from build123d import *

# Parameters (mm, degrees)
SKETCH1_R                 = 31.75
CENTERCIRCLEEXTRUDE_DEPTH = 19.558
SKETCH2_R                 = 80.01
BASEEXPAND_DEPTH          = 7.62
SKETCH3_R                 = 27.559
CENTERCUT_DEPTH           = 27.178
SKETCH4_R                 = 6.731
OUTERCIRCLECUT_DEPTH      = 7.62
SKETCH8_R                 = 80.01
STARFISHCUT_DEPTH         = 7.62
BATMAN_CUT_DEPTH          = 5.08
FILLET1_R                 = 2.54


with BuildPart() as part:
    # Sketch1 → CenterCircleExtrude (new body)
    with BuildSketch(Plane(origin=(0, 0, 0), x_dir=(1, 0, 0), z_dir=(0, 1, 0))):
        with Locations(Location((0, 0, 0), (0, 0, 270))):
            Circle(SKETCH1_R)
    extrude(amount=CENTERCIRCLEEXTRUDE_DEPTH)

    # Sketch2 → BaseExpand (add)
    with BuildSketch(Plane.XZ):
        with Locations(Location((0, 0, 0), (0, 0, 90))):
            Circle(SKETCH2_R)
    extrude(amount=BASEEXPAND_DEPTH)

    # Sketch3 → CenterCut (cut)
    with BuildSketch(Plane(origin=(0, 19.558, 0), x_dir=(1, 0, 0), z_dir=(0, 1, 0))):
        with Locations(Location((0, 0, 0), (0, 0, 270))):
            Circle(SKETCH3_R)
    extrude(amount=-CENTERCUT_DEPTH, mode=Mode.SUBTRACT)

    # Sketch4 → OuterCircleCut (cut)
    with BuildSketch(Plane(origin=(0, 0, 0), x_dir=(1, 0, 0), z_dir=(0, 1, 0))):
        with Locations(Location((-0.261130397, 55.117381423, 0), (0, 0, 270))):
            Circle(SKETCH4_R)
        with Locations(Location((47.602487304, 27.784836269, 0), (0, 0, 270))):
            Circle(SKETCH4_R)
        with Locations(Location((47.863617701, -27.332545154, 0), (0, 0, 270))):
            Circle(SKETCH4_R)
        with Locations(Location((0.261130397, -55.117381423, 0), (0, 0, 270))):
            Circle(SKETCH4_R)
        with Locations(Location((-47.602487304, -27.784836269, 0), (0, 0, 270))):
            Circle(SKETCH4_R)
        with Locations(Location((-47.863617701, 27.332545154, 0), (0, 0, 270))):
            Circle(SKETCH4_R)
    extrude(amount=-OUTERCIRCLECUT_DEPTH, mode=Mode.SUBTRACT)

    # Sketch8 → StarfishCut (cut)
    with BuildSketch(Plane(origin=(0, 0, 0), x_dir=(1, 0, 0), z_dir=(0, 1, 0))):
        Circle(SKETCH8_R)
        with BuildLine():
            ThreePointArc((-9.691634922, 58.167231466), (0, 65.278), (9.691634922, 58.167231466))
            ThreePointArc((9.691634922, 58.167231466), (14.680421474, 46.487646722), (20.366200635, 35.131036031))
            ThreePointArc((20.366200635, 35.131036031), (32.932591729, 35.888695551), (45.430991402, 37.398079103))
            ThreePointArc((45.430991402, 37.398079103), (46.084351809, 37.521062437), (46.744356679, 37.60105177))
            ThreePointArc((46.744356679, 37.60105177), (54.497784748, 34.973113956), (57.796096952, 27.480261323))
            ThreePointArc((57.796096952, 27.480261323), (57.324919213, 24.422104494), (55.95508845, 21.647596369))
            ThreePointArc((55.95508845, 21.647596369), (55.55581322, 21.116010052), (55.122626325, 20.611675009))
            ThreePointArc((55.122626325, 20.611675009), (47.502202506, 10.451466749), (40.509978727, -0.15086779))
            ThreePointArc((40.509978727, -0.15086779), (47.449326667, -10.654851952), (55.005691003, -20.7240918))
            ThreePointArc((55.005691003, -20.7240918), (55.438877898, -21.228426843), (55.838153128, -21.76001316))
            ThreePointArc((55.838153128, -21.76001316), (57.207983891, -24.534521285), (57.67916163, -27.592678114))
            ThreePointArc((57.67916163, -27.592678114), (54.380849426, -35.085530747), (46.627421357, -37.713468561))
            ThreePointArc((46.627421357, -37.713468561), (45.967416487, -37.633479228), (45.31405608, -37.510495894))
            ThreePointArc((45.31405608, -37.510495894), (32.70484571, -35.991119409), (20.026842771, -35.236843257))
            ThreePointArc((20.026842771, -35.236843257), (14.399799615, -46.498486939), (9.457764278, -58.077110338))
            ThreePointArc((9.457764278, -58.077110338), (9.237590766, -58.704428716), (8.976861126, -59.316004366))
            ThreePointArc((8.976861126, -59.316004366), (-0.233870644, -65.187878872), (-9.444602414, -59.316004366))
            ThreePointArc((-9.444602414, -59.316004366), (-9.705332054, -58.704428716), (-9.925505566, -58.077110338))
            ThreePointArc((-9.925505566, -58.077110338), (-14.914292118, -46.397525594), (-20.600071279, -35.040914903))
            ThreePointArc((-20.600071279, -35.040914903), (-33.166462373, -35.798574423), (-45.664862046, -37.307957975))
            ThreePointArc((-45.664862046, -37.307957975), (-46.318222453, -37.430941309), (-46.978227323, -37.510930642))
            ThreePointArc((-46.978227323, -37.510930642), (-56.668785698, -32.470140195), (-56.188959094, -21.557475241))
            ThreePointArc((-56.188959094, -21.557475241), (-55.789683864, -21.025888924), (-55.356496969, -20.521553881))
            ThreePointArc((-55.356496969, -20.521553881), (-47.73607315, -10.361345621), (-40.743849371, 0.240988918))
            ThreePointArc((-40.743849371, 0.240988918), (-47.683197311, 10.74497308), (-55.239561647, 20.814212928))
            ThreePointArc((-55.239561647, 20.814212928), (-55.672748542, 21.318547971), (-56.072023772, 21.850134288))
            ThreePointArc((-56.072023772, 21.850134288), (-56.551850376, 32.762799241), (-46.861292001, 37.803589689))
            ThreePointArc((-46.861292001, 37.803589689), (-46.201287131, 37.723600356), (-45.547926724, 37.600617021))
            ThreePointArc((-45.547926724, 37.600617021), (-32.938716354, 36.081240537), (-20.260713415, 35.326964385))
            ThreePointArc((-20.260713415, 35.326964385), (-14.633670259, 46.588608067), (-9.691634922, 58.167231466))
        make_face(mode=Mode.SUBTRACT)
    extrude(amount=-STARFISHCUT_DEPTH, mode=Mode.SUBTRACT)

    # Sketch14 → Batman Cut (cut)
    with BuildSketch(Plane(origin=(0, 0, 0), x_dir=(1, 0, 0), z_dir=(0, 1, 0))):
        with BuildLine():
            Line((35.018559386, 8.520826348), (24.742614343, 26.319285257))
            ThreePointArc((24.742614343, 26.319285257), (26.523552445, 32.965836738), (33.170103927, 31.184898636))
            Line((33.170103927, 31.184898636), (43.446048969, 13.386439727))
            ThreePointArc((43.446048969, 13.386439727), (41.665110867, 6.739888246), (35.018559386, 8.520826348))
        make_face()
        with BuildLine():
            Line((24.888531771, -26.066548858), (35.164476813, -8.268089949))
            ThreePointArc((35.164476813, -8.268089949), (41.811028295, -6.487151847), (43.591966397, -13.133703329))
            Line((43.591966397, -13.133703329), (33.316021354, -30.932162238))
            ThreePointArc((33.316021354, -30.932162238), (26.669469873, -32.71310034), (24.888531771, -26.066548858))
        make_face()
        with BuildLine():
            Line((-10.130027615, -34.587375206), (10.42186247, -34.587375206))
            ThreePointArc((10.42186247, -34.587375206), (15.28747585, -39.452988585), (10.42186247, -44.318601965))
            Line((10.42186247, -44.318601965), (-10.130027615, -44.318601965))
            ThreePointArc((-10.130027615, -44.318601965), (-14.995640994, -39.452988585), (-10.130027615, -34.587375206))
        make_face()
        with BuildLine():
            Line((10.130027615, 34.587375206), (-10.42186247, 34.587375206))
            ThreePointArc((-10.42186247, 34.587375206), (-15.28747585, 39.452988585), (-10.42186247, 44.318601965))
            Line((-10.42186247, 44.318601965), (10.130027615, 44.318601965))
            ThreePointArc((10.130027615, 44.318601965), (14.995640994, 39.452988585), (10.130027615, 34.587375206))
        make_face()
        with BuildLine():
            Line((-35.018559386, -8.520826348), (-24.742614343, -26.319285257))
            ThreePointArc((-24.742614343, -26.319285257), (-26.523552445, -32.965836738), (-33.170103927, -31.184898636))
            Line((-33.170103927, -31.184898636), (-43.446048969, -13.386439727))
            ThreePointArc((-43.446048969, -13.386439727), (-41.665110867, -6.739888246), (-35.018559386, -8.520826348))
        make_face()
        with BuildLine():
            Line((-24.888531771, 26.066548858), (-35.164476813, 8.268089949))
            ThreePointArc((-35.164476813, 8.268089949), (-41.811028295, 6.487151847), (-43.591966397, 13.133703329))
            Line((-43.591966397, 13.133703329), (-33.316021354, 30.932162238))
            ThreePointArc((-33.316021354, 30.932162238), (-26.669469873, 32.71310034), (-24.888531771, 26.066548858))
        make_face()
    extrude(amount=-BATMAN_CUT_DEPTH, mode=Mode.SUBTRACT)

    # Fillet1
    fillet1_edges = [part.edges().sort_by_distance(p)[0] for p in [
        (-20.260713415, -3.81, -35.326964385),
        (-40.743849371, -3.81, -0.240988918),
        (-20.600071279, -3.81, 35.040914903),
        (20.026842771, -3.81, 35.236843257),
        (40.509978727, -3.81, 0.15086779),
        (20.366200635, -3.81, -35.131036031),
    ]]
    fillet(fillet1_edges, radius=FILLET1_R)


solid = part.part
Source: CAD feature listing. Evaluate the final solid. Frame: model axes, mm. A direction names the side the tool comes from. Give positions to 0.01 mm unless a question says otherwise; leave off trailing zeros. Order: outer loops, then holes, each group sorted by start corner. A loop starts at its lowest first (then second) coordinate and runs counter-clockwise, first axis right, second up. Notation, with made-up numbers: (5, -8) -> (37, -8) arc R24 ccw to (37, 30) -> close; hole circle Ø10 at (-16.5, 32.5). An arc over 180 degrees is marked (long way). Write item = value, one per line.
Item 1: Section query C-C (x = -30). Output: boundary loops of the cut face in (y, z).
Check result:
outline = (-7.62, -35.84) -> (0, -35.84) -> (0, -33.28) -> (-5.08, -33.28) -> (-5.08, -17.21) -> (0, -17.21) -> (0, -10.4) -> (19.56, -10.4) -> (19.56, 10.4) -> (0, 10.4) -> (0, 17.21) -> (-5.08, 17.21) -> (-5.08, 33.5) -> (0, 33.5) -> (0, 35.54) -> (-7.62, 35.54) -> close
Item 2: Ray query, probe 1 along Y at (x, z) = (5, 34); probe 2 along X at (y, z) = (8.75, -18); probe 3 along Z at (x, y) = (2.5, -3.5). Return the intervals inside material, ascending.
Check result:
probe_1 = -7.62 to 0
probe_2 = -26.15 to -20.87, 20.87 to 26.15
probe_3 = -64.97 to -61.26, -48.98 to -44.32, -34.59 to -27.45, 27.45 to 34.59, 44.32 to 48.77, 61.47 to 64.81
Item 3: Set-up query: faces 1 (the face through (-15.286, -2.504, -39.346)), 2 (the face through (41.892, -3.757, 30.438)), 3 (the face through (33.66, -3.76, 36.08)). Return all of +Z, -Z, +X, -X, +Y, -Y with unobstructed straight access to the full face (end or side cutting, diameter ignored); none if empty.
Check result:
face_1 = +Y
face_2 = +Y, -Y
face_3 = +Z, +Y, -Y
Item 4: Section query B-B (z = -56.5). Output: boundary loops of the cut face in (x, y).
Check result:
outline = (-10.35, -7.62) -> (-6.85, -7.62) -> (-6.85, 0) -> (-10.35, 0) -> close; (6.33, -7.62) -> (10.35, -7.62) -> (10.35, 0) -> (6.33, 0) -> close
Item 5: Contact query for flat-ended pins moving along their axis: pin 1 (5 mm diameter, centred on x = 3, z = 41, fed in from +Y); pin 2 (10 mm diameter, centred on y = 1.5, z = 17.5, fed in from -X); pin 3 (21.5 mm diameter, centred on x = 0.26, z = 55.12, fed in from +Y). Output: stop coordinate, or through.
Check result:
pin_1 = -5.08
pin_2 = -56.65
pin_3 = 0
Item 6: Section query A-A (x = -17.5). Output: boundary loops of the cut face in (y, z), then the cut area to 3 significant figures.
Check result:
outline = (-7.62, -40.64) -> (0, -40.64) -> (0, -26.49) -> (19.56, -26.49) -> (19.56, -21.29) -> (-7.62, -21.29) -> close; (-7.62, 21.29) -> (19.56, 21.29) -> (19.56, 26.49) -> (0, 26.49) -> (0, 41.02) -> (-7.62, 41.02) -> close
area = 501 mm²
